Here's how the part is built. I have some questions about the finished solid (model axes, mm). A direction names the side the tool comes from. Coordinates: 2 decimals unless noted, no trailing zeros. Order: outer loops, then holes, each group sorted by start corner. A loop starts at its lowest first (then second) coordinate and runs counter-clockwise, first axis right, second up. Notation, with made-up numbers: (37.25, 33.5) - (82.25, 33.5) arc R22 ccw to (82.25, 57.5) - close; hole circle Ø1 at (-16.5, -40). An arc over 180 degrees is marked (long way). Answer in a Markdown table with one row per item. Add a question column.
Item 1: I want a section at B-B (x = 46.5). Please give me the cut outline in (y, z), plus the area to 3 significant figures.
Item 2: I want a section at A-A (y = 0). Please give me the cut outline in (x, z).
Item 3: Will these pins go through, and if not, where does the flat tip stop? pin 1 Ø1 at (x, y) = (7.5, -16.5) entering from +Z; pin 2 Ø1 at (x, z) = (25, 20.5) entering from +Y; pin 3 Ø3 at (x, y) = (47, -38) entering from +Z.
Item 4: On a 3-axis mill with a long thin cutter (end or side, diameter ignored), from which of +Z, -Z, +X, -X, +Y, -Y can I reach the whole of each face in a straight line? I mean faces 4 (the flat face through (50, 1, 28)), 5 (the flat face through (40, -32, 0)), 6 (the flat face through (30, -34, 10)). Say none if no direction works.
Item 5: I want a section at C-C (z = 0). Please give me the cut outline in (x, y).
Item 6: Thinking about a two-plate mould opening in Z: for faces 1 (the cylindrical face through (12.32, -29.97, -1.32)), 2 (the flat face through (50, 1, -23)), 3 (the cylindrical face through (25.35, 13.856, 5.745)), which applies, +Z half, -Z half, draft (parallel to the pull), parting line (faces both ways), or undercut?
Item 7: If I drill on line 1 along Z through (x, y) = (24, 0); line 2 along Z through (x, y) = (31, 0); line 3 along Y through (x, z) = (18, 0), over which ranges is the centre line in solid material (lowest first)? Write a range as from..to.
```python
from build123d import *

# Parameters (mm, degrees)
F2_W     = 110
F2_H     = 12
F3_DEPTH = 10
F4_W     = 6
F4_H     = 6
F5_DEPTH = 20
F6_R     = 5


with BuildPart() as f1:
    # F0 (on Top) → F1 (revolve)
    with BuildSketch(Plane.XY):
        Polygon((0, 30), (0, 15), (50, 15), (50, 50), (30, 50), (30, 30), align=None)
    revolve(axis=Axis((25, 0, 0), (-1, 0, 0)))

    # F2 (on face) → F3 (cut)
    with BuildSketch(Plane.YZ.offset(50)):
        Rectangle(F2_W, F2_H)
    extrude(amount=-F3_DEPTH, mode=Mode.SUBTRACT)

    # F4 (on face) → F5 (cut)
    with BuildSketch(Plane(origin=(0, 0, 0), x_dir=(0, -1, 0), z_dir=(-1, 0, 0))):
        with Locations((15, 0)):
            Rectangle(F4_W, F4_H)
    extrude(amount=-F5_DEPTH, mode=Mode.SUBTRACT)

    # F6
    f6_edges = [f1.edges().sort_by_distance(p)[0] for p in [
        (30, -30, 0),
    ]]
    fillet(f6_edges, radius=F6_R)


solid = f1.part
```
Values follow:
| question | item | result |
|---|---|---|
| 1 | outline | (-49.64, -6) arc R50 ccw to (49.64, -6) - (13.75, -6) arc R15 cw to (-13.75, -6) - close; (-49.64, 6) - (-13.75, 6) arc R15 cw to (13.75, 6) - (49.64, 6) arc R50 ccw to start |
| 1 | area | 6,300 mm^2 |
| 2 | outline | (0, -30) - (25, -30) arc R5 cw to (30, -35) - (30, -50) - (50, -50) - (50, -15) - (0, -15) - close; (0, 15) - (50, 15) - (50, 50) - (30, 50) - (30, 35) arc R5 cw to (25, 30) - (0, 30) - close |
| 3 | pin 1 | stops at z = 25.38 |
| 3 | pin 2 | stops at y = 22.36 |
| 3 | pin 3 | stops at z = 34.17 |
| 4 | face 4 | +Z, -Z, +X, +Y, -Y |
| 4 | face 5 | +X, +Y, -Y |
| 4 | face 6 | -X |
| 5 | outline | (0, -30) - (25, -30) arc R5 cw to (30, -35) - (30, -50) - (40, -50) - (40, -15) - (20, -15) - (20, -18) - (0, -18) - close; (0, 15) - (40, 15) - (40, 50) - (30, 50) - (30, 35) arc R5 cw to (25, 30) - (0, 30) - close |
| 6 | face 1 | parting line |
| 6 | face 2 | draft |
| 6 | face 3 | undercut |
| 7 | line 1 | z = -30..-15, 15..30 |
| 7 | line 2 | z = -50..-15, 15..50 |
| 7 | line 3 | y = -30..-18, 15..30 |
